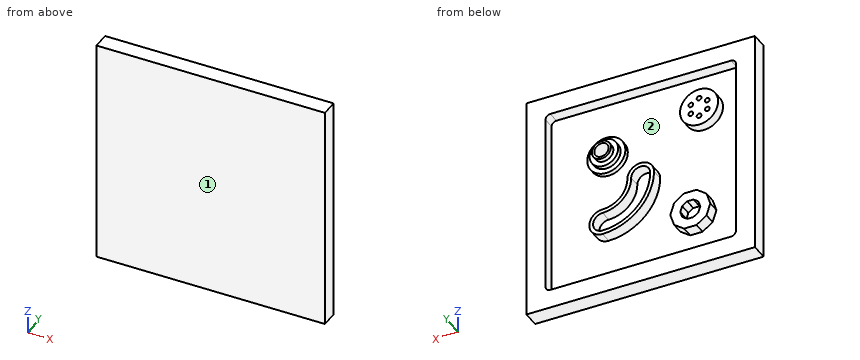
```python
from build123d import *

# Parameters (mm, degrees)
SKETCH1_W           = 152.4
SKETCH1_H           = 152.4
BOSS_EXTRUDE1_DEPTH = 11.1125
CUT_EXTRUDE1_DEPTH  = 7.9375
SKETCH3_R           = 12.7
BOSS_EXTRUDE2_DEPTH = 6.35
SKETCH4_R           = 1.5875
CUT_EXTRUDE2_DEPTH  = 6.35
BOSS_EXTRUDE3_DEPTH = 7.9375
EXTRUDE_THIN6_DEPTH = 7.9375
SKETCH8_R           = 12.7
BOSS_EXTRUDE4_DEPTH = 3.175
SKETCH9_R           = 9.525
BOSS_EXTRUDE5_DEPTH = 3.175
SKETCH10_R          = 6.35
BOSS_EXTRUDE6_DEPTH = 3.175
SKETCH11_R          = 4.7625
CUT_EXTRUDE3_DEPTH  = 10.16


with BuildPart() as part:
    # Sketch1 → Boss-Extrude1 (new body)
    with BuildSketch(Plane(origin=(0, 0, 0), x_dir=(1, 0, 0), z_dir=(0, 1, 0))):
        with Locations((76.2, 76.2)):
            Rectangle(SKETCH1_W, SKETCH1_H)
    extrude(amount=BOSS_EXTRUDE1_DEPTH)

    # Sketch2 → Cut-Extrude1 (cut)
    with BuildSketch(Plane(origin=(0, 11.1125, 0), x_dir=(1, 0, 0), z_dir=(0, 1, 0))):
        with BuildLine():
            Line((136.525, 139.7), (15.875, 139.7))
            ThreePointArc((15.875, 139.7), (13.62993597, 138.77006403), (12.7, 136.525))
            Line((12.7, 136.525), (12.7, 15.875))
            ThreePointArc((12.7, 15.875), (13.62993597, 13.62993597), (15.875, 12.7))
            Line((15.875, 12.7), (136.525, 12.7))
            ThreePointArc((136.525, 12.7), (138.77006403, 13.62993597), (139.7, 15.875))
            Line((139.7, 15.875), (139.7, 136.525))
            ThreePointArc((139.7, 136.525), (138.77006403, 138.77006403), (136.525, 139.7))
        make_face()
    extrude(amount=-CUT_EXTRUDE1_DEPTH, mode=Mode.SUBTRACT)

    # Sketch3 → Boss-Extrude2 (add)
    with BuildSketch(Plane(origin=(0, 3.175, 0), x_dir=(1, 0, 0), z_dir=(0, 1, 0))):
        with Locations(Location((38.1, 38.1, 0), (0, 0, 270))):
            Circle(SKETCH3_R)
    extrude(amount=BOSS_EXTRUDE2_DEPTH)

    # Sketch4 → Cut-Extrude2 (cut)
    with BuildSketch(Plane(origin=(0, 9.525, 0), x_dir=(1, 0, 0), z_dir=(0, 1, 0))):
        with Locations(Location((38.1, 44.45, 0), (0, 0, 270))):
            Circle(SKETCH4_R)
        with Locations(Location((43.599261314, 41.275, 0), (0, 0, 270))):
            Circle(SKETCH4_R)
        with Locations(Location((43.599261314, 34.925, 0), (0, 0, 270))):
            Circle(SKETCH4_R)
        with Locations(Location((38.1, 31.75, 0), (0, 0, 270))):
            Circle(SKETCH4_R)
        with Locations(Location((32.600738686, 34.925, 0), (0, 0, 270))):
            Circle(SKETCH4_R)
        with Locations(Location((32.600738686, 41.275, 0), (0, 0, 270))):
            Circle(SKETCH4_R)
    extrude(amount=-CUT_EXTRUDE2_DEPTH, mode=Mode.SUBTRACT)

    # Sketch5 → Boss-Extrude3 (add)
    with BuildSketch(Plane(origin=(0, 3.175, 0), x_dir=(1, 0, 0), z_dir=(0, 1, 0))):
        Polygon((53.918108532, 103.404018082), (56.468413513, 111.25304974), (53.918108532, 119.102081397), (47.241323408, 123.95304974), (38.988363123, 123.95304974), (32.311578, 119.102081397), (29.761273018, 111.25304974), (32.311578, 103.404018082), (38.988363123, 98.55304974), (47.241323408, 98.55304974), align=None)
        Polygon((49.79162839, 111.25304974), (48.516475899, 115.177565568), (45.178083337, 117.60304974), (41.051603195, 117.60304974), (37.713210633, 115.177565568), (36.438058142, 111.25304974), (37.713210633, 107.328533911), (41.051603195, 104.90304974), (45.178083337, 104.90304974), (48.516475899, 107.328533911), align=None, mode=Mode.SUBTRACT)
    extrude(amount=BOSS_EXTRUDE3_DEPTH)

    # Sketch6 → Extrude-Thin6 (add)
    with BuildSketch(Plane(origin=(0, 3.175, 0), x_dir=(1, 0, 0), z_dir=(0, 1, 0))):
        with BuildLine():
            ThreePointArc((101.6, 92.71), (89.925667043, 87.874332957), (85.09, 76.2))
            ThreePointArc((85.09, 76.2), (76.2, 67.31), (67.31, 76.2))
            ThreePointArc((67.31, 76.2), (77.353308473, 100.446691527), (101.6, 110.49))
            ThreePointArc((101.6, 110.49), (110.49, 101.6), (101.6, 92.71))
        make_face()
        with BuildLine():
            ThreePointArc((101.6, 95.25), (88.129615818, 89.670384182), (82.55, 76.2))
            ThreePointArc((82.55, 76.2), (76.2, 69.85), (69.85, 76.2))
            ThreePointArc((69.85, 76.2), (79.149359697, 98.650640303), (101.6, 107.95))
            ThreePointArc((101.6, 107.95), (107.95, 101.6), (101.6, 95.25))
        make_face(mode=Mode.SUBTRACT)
    extrude(amount=EXTRUDE_THIN6_DEPTH)

    # Sketch8 → Boss-Extrude4 (add)
    with BuildSketch(Plane(origin=(0, 3.175, 0), x_dir=(1, 0, 0), z_dir=(0, 1, 0))):
        with Locations(Location((101.6, 50.8, 0), (0, 0, 270))):
            Circle(SKETCH8_R)
    extrude(amount=BOSS_EXTRUDE4_DEPTH)

    # Sketch9 → Boss-Extrude5 (add)
    with BuildSketch(Plane(origin=(0, 6.35, 0), x_dir=(1, 0, 0), z_dir=(0, 1, 0))):
        with Locations(Location((101.6, 50.8, 0), (0, 0, 270))):
            Circle(SKETCH9_R)
    extrude(amount=BOSS_EXTRUDE5_DEPTH)

    # Sketch10 → Boss-Extrude6 (add)
    with BuildSketch(Plane(origin=(0, 9.525, 0), x_dir=(1, 0, 0), z_dir=(0, 1, 0))):
        with Locations(Location((101.6, 50.8, 0), (0, 0, 270))):
            Circle(SKETCH10_R)
    extrude(amount=BOSS_EXTRUDE6_DEPTH)

    # Sketch11 → Cut-Extrude3 (cut)
    with BuildSketch(Plane(origin=(0, 12.7, 0), x_dir=(1, 0, 0), z_dir=(0, 1, 0))):
        with Locations(Location((101.6, 50.8, 0), (0, 0, 270))):
            Circle(SKETCH11_R)
    extrude(amount=-CUT_EXTRUDE3_DEPTH, mode=Mode.SUBTRACT)


solid = part.part
```
Read the model definition and answer for the solid it produces. Units are mm, in the model's axes. Face numbers are marked on the shaded views. A direction names the side the tool comes from. Round coordinates to 2 decimals unless told otherwise and drop trailing zeros. Loops run counter-clockwise (first coordinate to the right, second up) from the corner with the lowest first, then second, coordinate; pieces in that order, holes last. Notation, with made-up numbers: (79.25, 8.5) -> (86.25, 8.5) arc R25 cw to (86.25, 23.5) -> close; hole circle Ø4 at (-29, 16.5). An arc over 180 degrees is marked (long way). One line per item, written item: value.
1) A cutting plane is placed at A-A (x = 118). Determine the outline of the cut face in (y, z) (1 decimal).
Answer list:
outline: (0, -152.4) -> (11.1, -152.4) -> (11.1, -139.7) -> (3.2, -139.7) -> (3.2, -12.7) -> (11.1, -12.7) -> (11.1, 0) -> (0, 0) -> close
2) A cutting plane is placed at B-B (z = -121.5). Determine the outline of the cut face in (x, y) (1 decimal), and give its area (3 significant figures).
Answer list:
outline: (0, 0) -> (152.4, 0) -> (152.4, 11.1) -> (139.7, 11.1) -> (139.7, 3.2) -> (50.6, 3.2) -> (50.6, 11.1) -> (35.6, 11.1) -> (35.6, 3.2) -> (12.7, 3.2) -> (12.7, 11.1) -> (0, 11.1) -> close
area: 805 mm²
3) Flat-ended cylindrical pins translate along their axes: P1, Ø21.5, axis at x = 98, z = -92.5, coming from the +Y side; P2, Ø3, axis at x = 43.6, z = -34.92, coming from the +Y side (3 decimals); P3, Ø3.5, axis at x = 44, z = -34.5, coming from the +Y side (3 decimals). Find the tip coordinate at first contact, or state that the pin passes through.
Answer list:
P1: stops at y = 11.11
P2: stops at y = 3.175
P3: stops at y = 9.525
4) For the marked faces 1 and 2, determine the directions among +Z, -Z, +X, -X, +Y, -Y from which every point of the face is accessible in a straight line to the end or side of a thin tool.
Answer list:
face 1: +Z, -Z, +X, -X, -Y
face 2: +Y
5) A cutting plane is placed at C-C (z = -73.5). Determine the outline of the cut face in (x, y) (1 decimal), and give its area (3 significant figures).
Answer list:
outline: (0, 0) -> (152.4, 0) -> (152.4, 11.1) -> (139.7, 11.1) -> (139.7, 3.2) -> (84.7, 3.2) -> (84.7, 11.1) -> (81.9, 11.1) -> (81.9, 3.2) -> (70.5, 3.2) -> (70.5, 11.1) -> (67.7, 11.1) -> (67.7, 3.2) -> (12.7, 3.2) -> (12.7, 11.1) -> (0, 11.1) -> close
area: 729 mm²
6) Consider L1, parallel to Z at x = 59.5, y = 11; L2, parallel to X at y = 4, z = -121; L3, parallel to Z at x = 77, y = 9. Determine where each line is inside the solid, lowest interval first. Write a range as [from, to].
Answer list:
L1: z = [-152.4, -139.7], [-12.7, 0]
L2: x = [0, 12.7], [34.92, 51.31], [139.7, 152.4]
L3: z = [-152.4, -139.7], [-100.09, -96.27], [-69.9, -67.35], [-12.7, 0]
